Source: CAD feature listing. Evaluate the final solid. Frame: model axes, mm. A direction names the side the tool comes from. Give positions to 0.01 mm unless a question says otherwise; leave off trailing zeros. Order: outer loops, then holes, each group sorted by start corner. A loop starts at its lowest first (then second) coordinate and runs counter-clockwise, first axis right, second up. Notation, with made-up numbers: M -19.75,-25.75 L 0.25,-25.75 A31 cw 0.25,13.25 Z; hole C 47,-24 d2. An arc over 180 degrees is marked long. Use CSV: the item, a comma, the result in double quotes. Start each with the question number.
1. Section query B-B, the plane z = -11. Return the cut outline in (x, y), plus the area to 3 significant figures.
2. Section query C-C, the plane y = -37. Return the cut outline in (x, z).
3. Mould query, pull axis Z, two halves, no side actions, for faces 4 (the conical face through (2.738, -4.624, 44.628)), 5 (the flat face through (5, -71, -41.24)), 6 (the cylindrical face through (5.01, -21.22, 107.5)). Classes: released by +Z, released by -Z, zero draft, split by the parting line, or undercut.
4. Section query D-D, the plane z = 80. Return the cut outline in (x, y), plus the area to 3 significant figures.
5. Pin query (flat end, axial travel): P1, Ø2, axis at x = 5.5, y = -53, coming from the +Z side; P2, Ø1.5, axis at x = 2, y = -37.5, coming from the +Z side; P3, Ø1.7, axis at x = 6.35, z = 116.24, coming from the +Y side. Return the tip coordinate at first contact, or that it passes through.
6. Reachability of faces 1 (the flat face through (5, -66.04, 36)), 2 (the flat face through (5, -76.2, 49)), 3 (the flat face through (5, -5, 0)) from +Z, -Z, +X, -X, +Y, -Y: full face, straight path, thin tool, end or side. Return the list, or none.
7. Section query A-A, the plane z = 17. Return the cut outline in (x, y), plus the area to 3 significant figures.
8. Line query: line 1 along Y through (x, z) = (6.25, 7.62); line 2 along Y through (x, z) = (8.5, 3); line 3 along Y through (x, z) = (8.25, 72). Output: solid intervals per line, ascending. Write a range as [from, to].
from build123d import *

# Parameters (mm, degrees)
BOSS_EXTRUDE1_DEPTH                               = 10.16
SKETCH2_R                                         = 1.4224
CUT_EXTRUDE2_DEPTH                                = 157.71111347
CUT_EXTRUDE3_REACH                                = 158.711
SKETCH3_R                                         = 1.4224
CSK_FOR_3_FLAT_HEAD_MACHINE_SCREW_100_D           = 2.794
CSK_FOR_3_FLAT_HEAD_MACHINE_SCREW_100_CSINK_D     = 7.7978
CSK_FOR_3_FLAT_HEAD_MACHINE_SCREW_100_CSINK_ANGLE = 82


with BuildPart() as part:
    # Sketch1 → Boss-Extrude1 (new body)
    with BuildSketch(Plane(origin=(0, 0, 0), x_dir=(0, 0, -1), z_dir=(1, 0, 0))):
        with BuildLine():
            Line((-136.560270522, -76.2), (41.239729478, -76.2))
            Line((41.239729478, -76.2), (41.239729478, -66.04))
            Line((41.239729478, -66.04), (-115.357986338, -66.04))
            ThreePointArc((-115.357986338, -66.04), (-120.636166121, -63.220342502), (-121.226894187, -57.265454545))
            ThreePointArc((-121.226894187, -57.265454545), (-93.164110025, -23.021842608), (-50.8, -10.16))
            Line((-50.8, -10.16), (0, -10.16))
            Line((0, -10.16), (0, 0))
            Line((0, 0), (-50.8, 0))
            ThreePointArc((-50.8, 0), (-108.161276136, -21.802013662), (-136.560270522, -76.2))
        make_face()
    extrude(amount=BOSS_EXTRUDE1_DEPTH)

    # Sketch2 → Cut-Extrude2 (cut, through all)
    with BuildSketch(Plane(origin=(10.16, 0, 0), x_dir=(0, 0, -1), z_dir=(1, 0, 0))):
        with Locations((-7.62, -5.08)):
            Circle(SKETCH2_R)
    extrude(amount=-CUT_EXTRUDE2_DEPTH, mode=Mode.SUBTRACT)

    # Sketch3 → Cut-Extrude3 (cut, up to next)
    with BuildSketch(Plane.XZ.offset(76.2), mode=Mode.PRIVATE) as cut_extrude3_sk1:
        with Locations(Location((6.35, 116.240270522, 0), (0, 0, 270))):
            Circle(SKETCH3_R)
    cut_extrude3_tool1 = extrude(cut_extrude3_sk1.sketch, amount=-CUT_EXTRUDE3_REACH, mode=Mode.PRIVATE) & part.part
    # Sketch3 → Cut-Extrude3 (cut, up to next)
    with BuildSketch(Plane.XZ.offset(76.2), mode=Mode.PRIVATE) as cut_extrude3_sk2:
        with Locations(Location((6.35, 65.440270522, 0), (0, 0, 270))):
            Circle(SKETCH3_R)
    cut_extrude3_tool2 = extrude(cut_extrude3_sk2.sketch, amount=-CUT_EXTRUDE3_REACH, mode=Mode.PRIVATE) & part.part
    add(cut_extrude3_tool1.solids().sort_by_distance((6.35, -76.2, 116.240271))[0], mode=Mode.SUBTRACT)
    add(cut_extrude3_tool2.solids().sort_by_distance((6.35, -76.2, 65.440271))[0], mode=Mode.SUBTRACT)

    # CSK for #3 Flat Head Machine Screw (100)1 (through all)
    with Locations(Plane.ZY):
        with Locations((7.62, -5.08)):
            csk_for_3_flat_head_machine_screw_100 = CounterSinkHole(CSK_FOR_3_FLAT_HEAD_MACHINE_SCREW_100_D / 2, CSK_FOR_3_FLAT_HEAD_MACHINE_SCREW_100_CSINK_D / 2, counter_sink_angle=CSK_FOR_3_FLAT_HEAD_MACHINE_SCREW_100_CSINK_ANGLE)

    # Mirror1: CSK for #3 Flat Head Machine Screw (100)1 across plane
    add(csk_for_3_flat_head_machine_screw_100.mirror(Plane(origin=(0, 0, 25.4), x_dir=(1, 0, 0), z_dir=(0, 0, -1))), mode=Mode.SUBTRACT)


solid = part.part
Result set:
1,outline,"M 0,-76.2 L 10.16,-76.2 L 10.16,-66.04 L 0,-66.04 Z"
1,area,"103 mm2"
2,outline,"M 0,108.85 L 10.16,108.85 L 10.16,121.66 L 0,121.66 Z"
3,face 4,"undercut"
3,face 5,"released by -Z"
3,face 6,"released by +Z"
4,outline,"M 0,-76.2 L 10.16,-76.2 L 10.16,-66.04 L 0,-66.04 Z; M 0,-15.98 L 10.16,-15.98 L 10.16,-5.09 L 0,-5.09 Z"
4,area,"214 mm2"
5,P1,"z = 130.87"
5,P2,"z = 122.52"
5,P3,"y = -29.03"
6,face 1,"-Z, +X, -X"
6,face 2,"+Z, -Z, +X, -X, -Y"
6,face 3,"-Z, +X, -X, +Y"
7,outline,"M 0,-76.2 L 10.16,-76.2 L 10.16,-66.04 L 0,-66.04 Z; M 0,-10.16 L 10.16,-10.16 L 10.16,0 L 0,0 Z"
7,area,"206 mm2"
8,line 1,"[-76.2, -66.04], [-10.16, -6.5], [-3.66, 0]"
8,line 2,"[-76.2, -66.04], [-10.16, 0]"
8,line 3,"[-76.2, -66.04], [-13.17, -2.64]"
